For this review, take the finished solid that the model builds, in its own axes (mm). A direction names the side the tool comes from. Round coordinates to 2 decimals unless told otherwise and drop trailing zeros. Order: outer loops, then holes, each group sorted by start corner. A loop starts at its lowest first (then second) coordinate and runs counter-clockwise, first axis right, second up. Notation, with made-up numbers: M -15.75,21.5 L -5.75,21.5 A31 cw -5.75,46.5 Z; hole C -36,-30.75 d3. An arc over 180 degrees is marked long. Write item = value, one per line. Start each with the question number.
from build123d import *

# Parameters (mm, degrees)
SKETCH1_W                       = 134.7
SKETCH1_H                       = 76.2
BOSS_EXTRUDE1_DEPTH             = 3
SKETCH2_W                       = 3
SKETCH2_H                       = 7.8
CUT_EXTRUDE1_DEPTH              = 78.437926754
LPATTERN1_COUNT                 = 4
LPATTERN1_PITCH                 = 22.8
F_3_0MM_CLEARANCE_DOWEL_HOLE1_D = 3
MIRROR4_COPY_1_SKETCH_W         = 3
MIRROR4_COPY_1_SKETCH_H         = 7.8
MIRROR4_COPY_1_DEPTH            = 78.437926754
MIRROR4_COPY_2_SKETCH_W         = 3
MIRROR4_COPY_2_SKETCH_H         = 7.8
MIRROR4_COPY_2_DEPTH            = 78.437926754
MIRROR4_COPY_3_SKETCH_W         = 3
MIRROR4_COPY_3_SKETCH_H         = 7.8
MIRROR4_COPY_3_DEPTH            = 78.437926754
SKETCH5_W                       = 7.8
SKETCH5_H                       = 3
BOSS_EXTRUDE2_DEPTH             = 3
LPATTERN2_COUNT                 = 5
LPATTERN2_PITCH                 = 22.8


with BuildPart() as part:
    # Sketch1 → Boss-Extrude1 (new body)
    with BuildSketch(Plane.XY):
        Rectangle(SKETCH1_W, SKETCH1_H)
    extrude(amount=BOSS_EXTRUDE1_DEPTH)

    # Sketch2 → Cut-Extrude1 (cut, through all)
    with BuildSketch(Plane.XY.offset(3)):
        with Locations((-65.85, 34.2)):
            Rectangle(SKETCH2_W, SKETCH2_H)
    cut_extrude1 = extrude(amount=-CUT_EXTRUDE1_DEPTH, mode=Mode.SUBTRACT)

    # LPattern1: Cut-Extrude1 ×4
    with Locations(*[(0, -i * LPATTERN1_PITCH, 0) for i in range(1, LPATTERN1_COUNT)]):
        add(cut_extrude1, mode=Mode.SUBTRACT)

    # Ø3.0mm Clearance Dowel Hole1 (through all)
    with Locations(Plane.XY.offset(3)):
        with Locations((-2.5, 0)):
            Hole(F_3_0MM_CLEARANCE_DOWEL_HOLE1_D / 2)

    # Mirror4: Cut-Extrude1 across plane
    add(cut_extrude1.mirror(Plane(origin=(0, 0, 0), x_dir=(0, 0, 1), z_dir=(1, 0, 0))), mode=Mode.SUBTRACT)

    # Mirror4 copy 1 sketch → Mirror4 copy 1 (cut, through all)
    with BuildSketch(Plane(origin=(0, -22.8, 3), x_dir=(-1, 0, 0), z_dir=(0, 0, 1))):
        with Locations((-65.85, -34.2)):
            Rectangle(MIRROR4_COPY_1_SKETCH_W, MIRROR4_COPY_1_SKETCH_H)
    extrude(amount=-MIRROR4_COPY_1_DEPTH, mode=Mode.SUBTRACT)

    # Mirror4 copy 2 sketch → Mirror4 copy 2 (cut, through all)
    with BuildSketch(Plane(origin=(0, -45.6, 3), x_dir=(-1, 0, 0), z_dir=(0, 0, 1))):
        with Locations((-65.85, -34.2)):
            Rectangle(MIRROR4_COPY_2_SKETCH_W, MIRROR4_COPY_2_SKETCH_H)
    extrude(amount=-MIRROR4_COPY_2_DEPTH, mode=Mode.SUBTRACT)

    # Mirror4 copy 3 sketch → Mirror4 copy 3 (cut, through all)
    with BuildSketch(Plane(origin=(0, -68.4, 3), x_dir=(-1, 0, 0), z_dir=(0, 0, 1))):
        with Locations((-65.85, -34.2)):
            Rectangle(MIRROR4_COPY_3_SKETCH_W, MIRROR4_COPY_3_SKETCH_H)
    extrude(amount=-MIRROR4_COPY_3_DEPTH, mode=Mode.SUBTRACT)

    # Sketch5 → Boss-Extrude2 (add)
    with BuildSketch(Plane(origin=(0, 38.1, 0), x_dir=(1, 0, 0), z_dir=(0, 1, 0))):
        with Locations((-47.65, -1.5)):
            Rectangle(SKETCH5_W, SKETCH5_H)
    boss_extrude2 = extrude(amount=BOSS_EXTRUDE2_DEPTH)

    # LPattern2: Boss-Extrude2 ×5
    with Locations(*[(i * LPATTERN2_PITCH, 0, 0) for i in range(1, LPATTERN2_COUNT)]):
        add(boss_extrude2)


solid = part.part
(1) We need section C-C, the plane y = 33. Write out the cut boundary in (x, z), then the cut area to 3 significant figures.
(2) For faces 1 (the flat face through (-51.55, 40, 2)), 2 (the flat face through (16.85, 40, 2)), 3 (the flat face through (-66, 15.3, 2)), 4 (the flat face through (-64.35, -34, 2)), 5 (the flat face through (66, -15.3, 2)), list the 3-axis set-ups (+Z, -Z, +X, -X, +Y, -Y) from which the entire face can be reached by the end or side of a thin tool; tool diameter is ignored.
(3) We need section A-A, the plane x = -2.5. Write out the cut boundary in (y, z), then the cut area to 3 significant figures.
(4) We need section D-D, the plane x = 14.5. Write out the cut boundary in (y, z), then the cut area to 3 significant figures.
(5) We need section B-B, the plane y = 0. Write out the cut boundary in (x, z), then the cut area to 3 significant figures.
(6) For line 1 along Y through (x, z) = (-2.5, 1.2); line 2 along Y through (x, z) = (48.5, 2.95); line 3 along X through (y, z) = (-12, 1.7), list the stretches that pass through material, from the lowest coordinate up.
(7) Draft analysis for pull direction Y (two halves, no side actions). For faces 6 (the flat face through (66, 15.3, 2)), 7 (the flat face through (-36, 38.1, 1)), 8 (the flat face through (-64.35, 34, 2)), state which applies: released by +Y, released by -Y, zero draft, split by the parting line, or undercut.
(8) Insertion check: pin 1 (1.5 mm diameter, centred on y = -12.5, z = 1, fed in from +X); pin 2 (1.5 mm diameter, centred on x = -15, z = 2, fed in from +Y); pin 3 (0.9 mm diameter, centred on x = 66.5, z = 1.5, fed in from -Y). Each pin has a flat end and moves straight along its axis. Give the tip position at first contact, or say it passes through.
Values:
q1.outline = M -64.35,0 L 64.35,0 L 64.35,3 L -64.35,3 Z
q1.area = 386 mm²
q2.face_1 = +Z, -Z, -X, +Y
q2.face_2 = +Z, -Z, +Y
q2.face_3 = +Z, -Z, -X
q2.face_4 = +Z, -Z, -X, -Y
q2.face_5 = +Z, -Z, +X
q3.outline = M -38.1,0 L -1.5,0 L -1.5,3 L -38.1,3 Z; M 1.5,0 L 41.1,0 L 41.1,3 L 1.5,3 Z
q3.area = 229 mm²
q4.outline = M -38.1,0 L 38.1,0 L 38.1,3 L -38.1,3 Z
q4.area = 229 mm²
q5.outline = M -67.35,0 L -4,0 L -4,3 L -67.35,3 Z; M -1,0 L 67.35,0 L 67.35,3 L -1,3 Z
q5.area = 395 mm²
q6.line_1 = -38.1 to -1.5, 1.5 to 41.1
q6.line_2 = -38.1 to 38.1
q6.line_3 = -64.35 to 64.35
q7.face_6 = undercut
q7.face_7 = released by +Y
q7.face_8 = zero draft
q8.pin_1 = 64.35
q8.pin_2 = 38.1
q8.pin_3 = -30.3
